Verification items for the finished model (mm, model axes). Face numbers are marked on the shaded views. A direction names the side the tool comes from. Round coordinates to 2 decimals unless told otherwise and drop trailing zeros. Write each loop counter-clockwise with the first axis right and the second up, starting at its lowest first coordinate (ties: lowest second). Pieces come first, ordered by that corner, then holes. Notation, with made-up numbers: (72.25, -38.5) - (77.25, -38.5) arc R26 ccw to (77.25, -8.5) - close; hole circle Ø10 at (23, 0). An arc over 180 degrees is marked (long way). Answer as a JSON object with one key per item and string values.
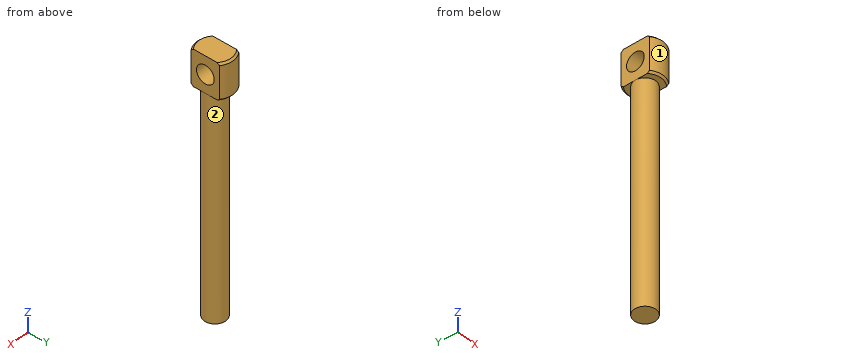
```python
from build123d import *

# Parameters (mm, degrees)
BOSS_EXTRUDE1_DEPTH = 10
SKETCH2_R           = 3
BOSS_EXTRUDE2_DEPTH = 61
CHAMFER1_SIZE       = 0.5
SKETCH3_R           = 2.5
CUT_EXTRUDE1_DEPTH  = 61


with BuildPart() as part:
    # Sketch1 → Boss-Extrude1 (new body)
    with BuildSketch(Plane.XY):
        with BuildLine():
            Line((3, 4), (3, -4))
            ThreePointArc((3, -4), (0, -5), (-3, -4))
            Line((-3, -4), (-3, 4))
            ThreePointArc((-3, 4), (0, 5), (3, 4))
        make_face()
    extrude(amount=-BOSS_EXTRUDE1_DEPTH)

    # Sketch2 → Boss-Extrude2 (add)
    with BuildSketch(Plane(origin=(0, 0, -10), x_dir=(-1, 0, 0), z_dir=(0, 0, -1))):
        Circle(SKETCH2_R)
    extrude(amount=BOSS_EXTRUDE2_DEPTH)

    # Chamfer1
    chamfer1_edges = [part.edges().sort_by_distance(p)[0] for p in [
        (0, -5, -10),
        (0, 5, -10),
        (0, -5, 0),
        (0, 5, 0),
    ]]
    chamfer(chamfer1_edges, length=CHAMFER1_SIZE)

    # Sketch3 → Cut-Extrude1 (cut)
    with BuildSketch(Plane.ZY.offset(3)):
        with Locations((-5, 0)):
            Circle(SKETCH3_R)
    extrude(amount=-CUT_EXTRUDE1_DEPTH, mode=Mode.SUBTRACT)


solid = part.part
```
Q1. Section check B-B, the plane x = 0. Record the cut outline in (y, z), then the cut area to 3 significant figures.
Geometry check:
{"outline": "(-5, -9.5) - (-4.5, -10) - (-3, -10) - (-3, -71) - (3, -71) - (3, -10) - (4.5, -10) - (5, -9.5) - (5, -0.5) - (4.5, 0) - (-4.5, 0) - (-5, -0.5) - close; hole circle Ø5 at (0, -5)", "area": "446 mm2"}
Q2. Section check D-D, the plane z = -58.5. Record the cut outline in (x, y).
Geometry check:
{"outline": "circle Ø6 at (0, 0)"}
Q3. Gauge pin test, flat ends, axial feed: P1, Ø4.5, axis at y = 0, z = -5, coming from the -X side; P2, Ø3, axis at y = 3, z = -34.5, coming from the -X side; P3, Ø2, axis at x = 1, z = -24.5, coming from the +Y side; P4, Ø2, axis at y = 3.5, z = -28, coming from the -X side. Record the tip position at first contact, or that the pin passes through.
Geometry check:
{"P1": "passes through", "P2": "stops at x = -2.6", "P3": "stops at y = 3", "P4": "stops at x = -1.66"}
Q4. Set-up check for the marked faces 1 and 2: record each of +Z, -Z, +X, -X, +Y, -Y from which the full face is reachable in a straight line by a thin tool's end or side.
Geometry check:
{"face 1": "+Z, -Z, -Y", "face 2": "-Z"}
Q5. Material ranges on line 1 along Z through (x, y) = (1.75, -3.5); line 2 along Y through (x, z) = (-0.75, -3.5); line 3 along Y through (x, z) = (0.25, -41), recorded low to high. Write a range as [from, to].
Geometry check:
{"line 1": "z = [-10, 0]", "line 2": "y = [-4.94, -2], [2, 4.94]", "line 3": "y = [-2.99, 2.99]"}
Q6. Section check A-A, the plane y = -1.25. Record the cut outline in (x, z), then the cut area to 3 significant figures.
Geometry check:
{"outline": "(-3, -10) - (-2.73, -10) - (-2.73, -71) - (2.73, -71) - (2.73, -10) - (3, -10) - (3, -7.17) - (-3, -7.17) - close; (-3, -2.83) - (3, -2.83) - (3, 0) - (-3, 0) - close", "area": "367 mm2"}
Q7. Section check C-C, the plane z = -5. Record the cut outline in (x, y).
Geometry check:
{"outline": "(-3, -4) arc R5 ccw to (3, -4) - (3, -2.5) - (-3, -2.5) - close; (-3, 2.5) - (3, 2.5) - (3, 4) arc R5 ccw to (-3, 4) - close"}
